Geometry check sheet. Reference: the model listing, model coordinates, mm. A direction names the side the tool comes from. Coordinates: 2 decimals unless noted, no trailing zeros. Loops run counter-clockwise (first coordinate to the right, second up) from the corner with the lowest first, then second, coordinate; pieces in that order, holes last. Notation, with made-up numbers: M 54.5,55.5 L 72.5,55.5 A25 cw 72.5,76.5 Z; hole C 12,11 d10. An arc over 180 degrees is marked long. Use CSV: the item, a comma, the result in double quotes.
```python
from build123d import *

# Parameters (mm, degrees)
CUT_EXTRUDE_12_DEPTH      = 102.948516419
CUT_EXTRUDE_12_DEPTH_BACK = 102.948516419
CUT_EXTRUDE_START         = 61
CUT_EXTRUDE_5_R0_25_DEPTH = 31


with BuildPart() as part:
    # Эскиз1 → Revolve 238 (revolve)
    with BuildSketch(Plane.XY, mode=Mode.PRIVATE) as revolve_238_sk:
        with BuildLine():
            Line((0, 32.5), (37, 32.5))
            Line((37, 32.5), (64.745695, 25.068113))
            ThreePointArc((64.745695, 25.068113), (65.002224223, 25.017098236), (65.263217049, 24.999995817))
            Line((65.263217049, 24.999995817), (69.749999449, 24.999995817))
            Line((69.749999449, 24.999995817), (70.749999449, 23.999995817))
            Line((70.749999449, 23.999995817), (70.749999449, 19.499995817))
            Line((70.749999449, 19.499995817), (79.25, 19.499995817))
            Line((79.25, 19.499995817), (79.25, 24))
            Line((79.25, 24), (80.25, 25))
            Line((80.25, 25), (88, 25))
            Line((88, 25), (91, 22))
            Line((91, 22), (91, 11))
            Line((91, 11), (90, 10))
            Line((90, 10), (61, 10))
            Line((61, 10), (61, 19))
            ThreePointArc((61, 19), (60.707106781, 19.707106781), (60, 20))
            Line((60, 20), (25, 20))
            Line((25, 20), (25, 27.1))
            ThreePointArc((25, 27.1), (24.882842712, 27.382842712), (24.6, 27.5))
            Line((24.6, 27.5), (0, 27.5))
            Line((0, 27.5), (0, 32.5))
        make_face()
    revolve(revolve_238_sk.sketch.rotate(Axis((0, 0, 0), (1, 0, 0)), 90), axis=Axis((0, 0, 0), (1, 0, 0)))

    # Эскиз2 → Наклон торца 12 градусов (cut, two sides: drawn at the far end of the back side and taken through both)
    with BuildSketch(Plane(origin=(0, 0, 0), x_dir=(1, 0, 0), z_dir=(0, 1, 0)).offset(-CUT_EXTRUDE_12_DEPTH_BACK)):
        Polygon((-25, 50), (15.30407244, 50), (-5.951583727, -50), (-25, -50), align=None)
    extrude(amount=CUT_EXTRUDE_12_DEPTH + CUT_EXTRUDE_12_DEPTH_BACK, mode=Mode.SUBTRACT)

    # Эскиз3 → Паз 5 R0.25 (cut)
    with BuildSketch(Plane(origin=(0, 0, 0), x_dir=(0, 0, -1), z_dir=(1, 0, 0)).offset(CUT_EXTRUDE_START)):
        with BuildLine():
            Line((0, -2.5), (0, 2.5))
            Line((0, 2.5), (-12.05, 2.5))
            ThreePointArc((-12.05, 2.5), (-12.226776695, 2.426776695), (-12.3, 2.25))
            Line((-12.3, 2.25), (-12.3, -2.25))
            ThreePointArc((-12.3, -2.25), (-12.226776695, -2.426776695), (-12.05, -2.5))
            Line((-12.05, -2.5), (0, -2.5))
        make_face()
    extrude(amount=CUT_EXTRUDE_5_R0_25_DEPTH, mode=Mode.SUBTRACT)


solid = part.part
```
1. Set-up check for faces 5 (the conical face through (90.16, -0.41, -10.15)), 6 (the flat face through (25, 18, 10)), 7 (the flat face through (76, -2.5, 11)), 8 (the flat face through (70.75, -20, 0)): record each of +Z, -Z, +X, -X, +Y, -Y from which the full face is reachable in a straight line by a thin tool's end or side.
The answers:
face 5,"+X"
face 6,"-X"
face 7,"+X, -X"
face 8,"none"
2. Gauge pin test, flat ends, axial feed: P1, Ø1.9, axis at x = 75, z = 11.5, coming from the +Y side; P2, Ø11.5, axis at y = 2.5, z = 7, coming from the -X side; P3, Ø1, axis at x = 75.5, z = -4.5, coming from the +Y side. Record the tip position at first contact, or that the pin passes through.
The answers:
P1,"y = 16.4"
P2,"x = 61"
P3,"y = 19.09"
3. Thickness scan on line 1 (Y direction, x = 12, z = 0); line 2 (Y direction, x = 49, z = 0); line 3 (Z direction, x = 49, y = -5). Record the ranges inside material, lowest first. Write a range as [from, to].
The answers:
line 1,"[-32.5, -27.5], [27.5, 32.5]"
line 2,"[-29.29, -20], [20, 29.29]"
line 3,"[-28.86, -19.36], [19.36, 28.86]"
4. Release check for a two-part mould opening along Y. For faces 1 (the flat face through (76, 0, 12.3)), 2 (the cylindrical face through (14.861, 10.533, 25.403)), 3 (the flat face through (79.25, -20, 0)), 4 (the cylindrical face through (18.76, -9.76, 31)) record: +Y half, -Y half, draft (parallel to the pull), parting line (faces both ways), or undercut.
The answers:
face 1,"undercut"
face 2,"undercut"
face 3,"draft"
face 4,"parting line"
5. Section check B-B, the plane x = 49.5. Record the cut outline in (y, z), plus the area to 3 significant figures.
The answers:
outline,"C 0,0 d58.3; hole C 0,0 d40"
area,"1,410 mm^2"
6. Section check A-A, the plane x = 68. Record the cut outline in (y, z).
The answers:
outline,"C 0,0 d50; hole M -2.5,9.68 A10 ccw long 2.5,9.68 L 2.5,12.05 A0.25 ccw 2.25,12.3 L -2.25,12.3 A0.25 ccw -2.5,12.05 Z"
